Here's how the part is built. I have some questions about the finished solid (model axes, mm). A direction names the side the tool comes from. Coordinates: 2 decimals unless noted, no trailing zeros. Write each loop counter-clockwise with the first axis right and the second up, starting at its lowest first coordinate (ties: lowest second). Pieces come first, ordered by that corner, then holes. Notation, with made-up numbers: (64, 22.25) - (107, 22.25) arc R17 ccw to (107, 31.25) - close; hole circle Ø2 at (-0.75, -37.5). An arc over 180 degrees is marked (long way). Answer in a Markdown table with one row per item. Add a question column.
Item 1: Imagine slicing it at D-D (y = 3). Please give me the cut outline in (x, z), plus the area to 3 significant figures.
Item 2: Imagine slicing it at B-B (y = -12). Please give me the cut outline in (x, z).
Item 3: We'd pull the mould along Y, two halves only. Please class faces 4 (the face through (0, -13.1, -35)), 5 (the face through (0, 17.379, -35)), 6 (the face through (-0.15, -21.507, -34.972)): +Y half, -Y half, draft (parallel to the pull), parting line (faces both ways), or undercut.
Item 4: Imagine slicing it at C-C (x = -1). Please give me the cut outline in (y, z).
Item 5: Which directions (+Z, -Z, +X, -X, +Y, -Y) give clear straight access to the entire face, cutting with the end or side of a thin tool? Please do faces 1 (the face through (0, 4, -34.5)), 2 (the face through (19.093, 9.844, -34.528)), 3 (the face through (7, -2.9, -35)).
Item 6: If I drill on probe 1 along X at (y, z) = (-7, -36.2); probe 2 along X at (y, z) = (2, -33.1); probe 3 along X at (y, z) = (-2.5, -34.2), over which ranges is the centre line in solid material (lowest first)? Write a range as from..to.
Item 7: I'm going to push flat-ended pins straight in: pin 1 (0.6 mm diameter, centred on y = -5, z = -34, fed in from +X); pin 2 (1.1 mm diameter, centred on x = -1.5, z = -35, fed in from -Y); pin 3 (6.5 mm diameter, centred on x = -0.5, y = 9, fed in from +Z); pin 4 (3 mm diameter, centred on x = 0.5, y = -17, fed in from +Z). Where does each tip first touch, or does it pass through?
Item 8: Imagine slicing it at A-A (z = -35.15). Please give me the cut outline in (x, y), plus the area to 3 significant figures.
from build123d import *

# Parameters (mm, degrees)
BOSS_EXTRUDE1_START = -36.5
BOSS_EXTRUDE1_DEPTH = 4
CUT_EXTRUDE1_START  = -21.50833
SKETCH2_W           = 6
SKETCH2_H           = 3
CUT_EXTRUDE1_DEPTH  = 38.387495
CUT_EXTRUDE2_DEPTH  = 2.2


with BuildPart() as part:
    # Sketch1 → Boss-Extrude1 (new body)
    with BuildSketch(Plane.XY.offset(BOSS_EXTRUDE1_START)):
        with BuildLine():
            Line((-2.043305467, 17.379165125), (-11.512304293, 15.726530305))
            ThreePointArc((-11.512304293, 15.726530305), (-19.035877705, 9.969093149), (-18.626760389, 0.504165125))
            Line((-18.626760389, 0.504165125), (-8.876760389, -16.383330249))
            ThreePointArc((-8.876760389, -16.383330249), (0, -21.508330249), (8.876760389, -16.383330249))
            Line((8.876760389, -16.383330249), (18.626760389, 0.504165125))
            ThreePointArc((18.626760389, 0.504165125), (19.035877705, 9.969093149), (11.512304293, 15.726530305))
            Line((11.512304293, 15.726530305), (2.043305467, 17.379165125))
            Line((2.043305467, 17.379165125), (-2.043305467, 17.379165125))
        make_face()
    extrude(amount=BOSS_EXTRUDE1_DEPTH)

    # Sketch2 → Cut-Extrude1 (cut)
    with BuildSketch(Plane(origin=(0, 0, 0), x_dir=(1, 0, 0), z_dir=(0, 1, 0)).offset(CUT_EXTRUDE1_START)):
        with Locations((0, 33)):
            Rectangle(SKETCH2_W, SKETCH2_H)
    extrude(amount=CUT_EXTRUDE1_DEPTH, mode=Mode.SUBTRACT)

    # Sketch4 → Cut-Extrude2 (cut)
    with BuildSketch(Plane(origin=(0, 0, -36.5), x_dir=(-1, 0, 0), z_dir=(0, 0, -1))):
        Polygon((-9.1, -2.9), (-9.1, -13.1), (9.1, -13.1), (9.1, -2.9), (4.9, -2.9), (4.9, -7.9), (-4.9, -7.9), (-4.9, -2.9), align=None)
    extrude(amount=-CUT_EXTRUDE2_DEPTH, mode=Mode.SUBTRACT)


solid = part.part
Here are the results:
| question | item | result |
|---|---|---|
| 1 | outline | (-19.66, -36.5) - (19.66, -36.5) - (19.66, -32.5) - (3, -32.5) - (3, -34.5) - (-3, -34.5) - (-3, -32.5) - (-19.66, -32.5) - close |
| 1 | area | 145 mm2 |
| 2 | outline | (-11.41, -36.5) - (-9.1, -36.5) - (-9.1, -34.3) - (-3, -34.3) - (-3, -32.5) - (-11.41, -32.5) - close; (3, -34.3) - (9.1, -34.3) - (9.1, -36.5) - (11.41, -36.5) - (11.41, -32.5) - (3, -32.5) - close |
| 3 | face 4 | undercut |
| 3 | face 5 | +Y half |
| 3 | face 6 | -Y half |
| 4 | outline | (-21.46, -36.5) - (-13.1, -36.5) - (-13.1, -34.5) - (-21.46, -34.5) - close; (-7.9, -36.5) - (17.38, -36.5) - (17.38, -32.5) - (16.88, -32.5) - (16.88, -34.5) - (-7.9, -34.5) - close |
| 5 | face 1 | +Z, -Y |
| 5 | face 2 | +Z, -Z, +X |
| 5 | face 3 | -Z |
| 6 | probe 1 | x = -14.29..-9.1, -4.9..4.9, 9.1..14.29 |
| 6 | probe 2 | x = -19.34..-3, 3..19.34 |
| 6 | probe 3 | x = -16.89..-3, 3..16.89 |
| 7 | pin 1 | stops at x = 15.62 |
| 7 | pin 2 | stops at y = -21.46 |
| 7 | pin 3 | stops at z = -32.5 |
| 7 | pin 4 | stops at z = -34.5 |
| 8 | outline | (-18.63, 0.5) - (-8.88, -16.38) arc R10.25 ccw to (8.88, -16.38) - (18.63, 0.5) arc R10.25 ccw to (11.51, 15.73) - (2.04, 17.38) - (-2.04, 17.38) - (-11.51, 15.73) arc R10.25 ccw to start; hole (-9.1, -13.1) - (9.1, -13.1) - (9.1, -2.9) - (4.9, -2.9) - (4.9, -7.9) - (-4.9, -7.9) - (-4.9, -2.9) - (-9.1, -2.9) - close |
| 8 | area | 977 mm2 |
